The listing builds one solid part. Answer for the finished solid, in the listing's coordinates (mm). A direction names the side the tool comes from. Give positions to 0.01 mm unless a question says otherwise; leave off trailing zeros. Loops run counter-clockwise (first coordinate to the right, second up) from the corner with the lowest first, then second, coordinate; pieces in that order, holes last. Notation, with made-up numbers: (53.5, 78) - (83.5, 78) arc R9 ccw to (83.5, 83) - close; hole circle Ø10 at (39.5, -38.75). An arc over 180 degrees is marked (long way). Answer in a Markdown table with one row per item. Add a question column.
Solid Edge part; units mm, degrees
sketch "Sketch1" plane through (0, 0, 0) normal (0, -1, 0) x (1, 0, 0)
  line L0 (280, 0) -> (280, 140)
  line L1 (0, 0) -> (280, 0)
  line L2 (0, 140) -> (0, 0)
  arc A0 (0, 140) -> (280, 140) centre (140, 140) cw
extrude "Protrusion1" add sketch "Sketch1" against normal blind 60
shell "Thinwall_1" thickness 10 removed faces 2 at (49.4667, 0, 236.1333) at (49.4667, 60, 236.1333)
fillet "Round_6" radius 5 1 edges at (270, 30, 10)
fillet "Round_7" radius 5 1 edges at (280, 30, 0)
fillet "Round_8" radius 5 1 edges at (0, 30, 0)
fillet "Round_9" radius 5 1 edges at (10, 30, 10)
sketch "Sketch2" plane through (140, 0, 140) normal (0, -1, 0) x (1, 0, 0)
  circle A0 centre (-40, -135) radius 2.5
  circle A1 centre (-110, -135) radius 2
  circle A2 centre (40, -135) radius 2.5
  circle A3 centre (110, -135) radius 2.5
extrude "ExtrudedProtrusion_18" add sketch "Sketch2" along normal blind 5
sketch "Sketch3" plane through (140, 60, 140) normal (0, -1, 0) x (1, 0, 0)
  circle A0 centre (-110, -135) radius 2.5
  circle A1 centre (-40, -135) radius 2.5
  circle A2 centre (40, -135) radius 2.5
  circle A3 centre (110, -135) radius 2.5
extrude "Cutout1" cut sketch "Sketch3" along normal blind 5
sketch "Sketch4" plane through (140, 0, 140) normal (0, -1, 0) x (1, 0, 0)
  circle A0 centre (-135, -80) radius 2.5
  circle A1 centre (-135, -10) radius 2.5
  circle A2 centre (135, -10) radius 2.5
  circle A3 centre (135, -80) radius 2.5
extrude "ExtrudedProtrusion_20" add sketch "Sketch4" along normal blind 5
sketch "Sketch5" plane through (140, 0, 140) normal (0, -1, 0) x (1, 0, 0)
  circle A0 centre (0, 135) radius 2.5
extrude "ExtrudedProtrusion_21" add sketch "Sketch5" along normal blind 5
sketch "Sketch6" plane through (140, 60, 140) normal (0, -1, 0) x (1, 0, 0)
  circle A0 centre (0, 135) radius 2.5
extrude "ExtrudedCutout_5" cut sketch "Sketch6" along normal blind 5
(1) Given pin 1 Ø1.5 at (x, z) = (179, 4) entering from +Y; pin 2 Ø8 at (x, z) = (46, 251) entering from +Y; pin 3 Ø3 at (y, z) = (48, 220.5) entering from +X, each flat-ended and moving along its own axis, determine where each tip first touches the part or whether it passes through.
(2) A tool of negligible diameter and unlimited length cuts with its end or side. For faces 5 (the face through (10, 30, 78)), 6 (the face through (141, 0, 6)), 7 (the face through (0, 30, 73)), from which of +Z, -Z, +X, -X, +Y, -Y can it reach the whole face along a straight path? Write none if from no direction.
(3) Find the intervals of material crossed by line 1 along Z through (x, y) = (140, 57); line 2 along X through (y, z) = (28, 135.5); line 3 along Z through (x, y) = (180, 57.2), in increasing order. Write a range as [from, to].
(4) A cutting plane is placed at A-A on z = 89. Determine the outline of the cut face in (x, y).
(5) A cutting plane is placed at B-B on y = 46.5. Determine the outline of the cut face in (x, z).
(6) A cutting plane is placed at C-C on x = 244. Determine the outline of the cut face in (y, z).
(7) The mould has two halves that part along Z. Classify faces 1 (the face through (143.079, 29.58, 279.966)), 2 (the face through (141, 60, 6)), 3 (the face through (142.86, 29.58, 269.97)), 4 (the face through (270, 30, 77)): pulls with the +Z half, pulls with the -Z half, needs draft (parallel to the pull), parting line crosses it, or undercut.
Evaluation:
| question | item | result |
|---|---|---|
| 1 | pin 1 | stops at y = 55 |
| 1 | pin 2 | passes through |
| 1 | pin 3 | stops at x = 255.58 |
| 2 | face 5 | +Y, -Y |
| 2 | face 6 | -Y |
| 2 | face 7 | +Z, -Z, -X, +Y, -Y |
| 3 | line 1 | z = [0, 10], [270, 272.5], [277.5, 280] |
| 3 | line 2 | x = [0, 10], [270, 280] |
| 3 | line 3 | z = [0, 2.5], [7.5, 10], [263.69, 274.16] |
| 4 | outline | (0, 0) - (10, 0) - (10, 60) - (0, 60) - close; (270, 0) - (280, 0) - (280, 60) - (270, 60) - close |
| 5 | outline | (0, 5) arc R5 ccw to (5, 0) - (275, 0) arc R5 ccw to (280, 5) - (280, 140) arc R140 ccw to (0, 140) - close; hole (10, 15) arc R5 ccw to (15, 10) - (265, 10) arc R5 ccw to (270, 15) - (270, 140) arc R130 ccw to (10, 140) - close |
| 6 | outline | (0, 0) - (60, 0) - (60, 10) - (0, 10) - close; (0, 218) - (60, 218) - (60, 233.72) - (0, 233.72) - close |
| 7 | face 1 | pulls with the +Z half |
| 7 | face 2 | needs draft |
| 7 | face 3 | undercut |
| 7 | face 4 | undercut |
